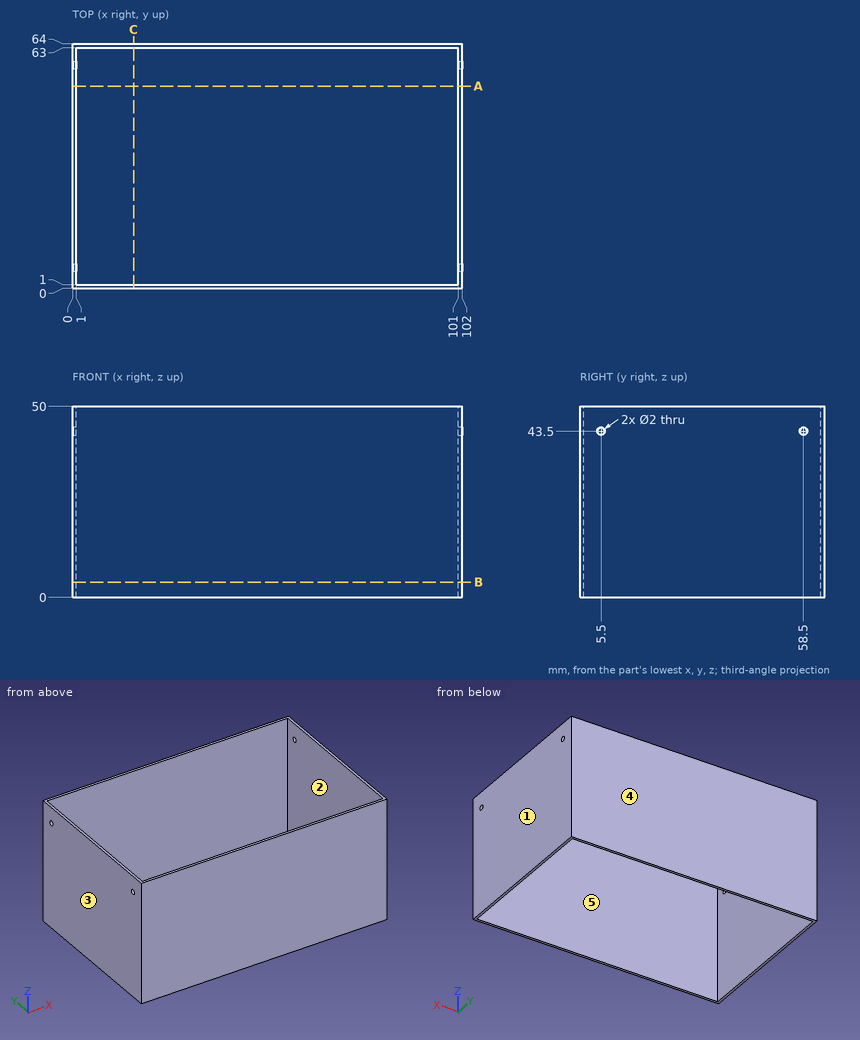
Input: dimensioned drawing with shaded views. Units: mm. Origin: part minimum x, y, z. A direction names the side the tool comes from. Give positions to 0.01 mm unless a question says otherwise; leave off trailing zeros. Loops run counter-clockwise (first coordinate to the right, second up) from the corner with the lowest first, then second, coordinate; pieces in that order, holes last. Notation, with made-up numbers: M 75.25,31 L 113.25,31 A23 cw 113.25,40 Z; hole C 45.5,-38 d7. An arc over 180 degrees is marked long. Put each result on its own line as item: value.
1) Cut plane A-A, the plane y = 53. Return the cut outline in (x, z), plus the area to 3 significant figures.
Computed values:
outline: M 0,0 L 1,0 L 1,50 L 0,50 Z; M 101,0 L 102,0 L 102,50 L 101,50 Z
area: 100 mm^2
2) Cut plane C-C, the plane x = 16. Return the cut outline in (y, z), plus the area to 3 significant figures.
Computed values:
outline: M 0,0 L 1,0 L 1,50 L 0,50 Z; M 63,0 L 64,0 L 64,50 L 63,50 Z
area: 100 mm^2
3) Cut plane B-B, the plane z = 4. Return the cut outline in (x, y), plus the area to 3 significant figures.
Computed values:
outline: M 0,0 L 102,0 L 102,64 L 0,64 Z; hole M 1,1 L 101,1 L 101,63 L 1,63 Z
area: 328 mm^2
4) Reachability of the marked faces 4 and 5 from +Z, -Z, +X, -X, +Y, -Y: full face, straight path, thin tool, end or side. Return the list, or none.
Computed values:
face 4: +Z, -Z, +X, -X, +Y
face 5: +Z, -Z
5) Material intervals for L1, parallel to Y at x = 0.5, z = 43.5; L2, parallel to Y at x = 5.5, z = 29; L3, parallel to X at y = 4, z = 47, sorted ascending. Write a range as from..to.
Computed values:
L1: y = 0..4.5, 6.5..57.5, 59.5..64
L2: y = 0..1, 63..64
L3: x = 0..1, 101..102
6) Mould query, pull axis X, two halves, no side actions, for the marked faces 1, 2 and 3. Classes: released by +X, released by -X, zero draft, split by the parting line, or undercut.
Computed values:
face 1: released by +X
face 2: undercut
face 3: released by -X
